Read the model definition and answer for the solid it produces. Units are mm, in the model's axes. A direction names the side the tool comes from. Coordinates: 2 decimals unless noted, no trailing zeros. Write each loop counter-clockwise with the first axis right and the second up, starting at its lowest first coordinate (ties: lowest second). Pieces come first, ordered by that corner, then holes. Notation, with made-up numbers: (67, 28) -> (102, 28) arc R27 ccw to (102, 54) -> close; hole circle Ø3 at (7, 24.25). An arc over 180 degrees is marked (long way). Return JSON: item names as keys, results as strings.
from build123d import *

# Parameters (mm, degrees)
BOSS_EXTRUDE1_DEPTH                     = 55
SHELL1_T                                = -3
CUT_EXTRUDE1_DEPTH                      = 2
BATTERY_CONNECTOR_SKETCH_3_R            = 2.15
CUT_EXTRUDE2_DEPTH                      = 3
BATTERY_CONNECTOR_SKETCH_4_R            = 2.15
CUT_EXTRUDE3_DEPTH                      = 3
BOSS_EXTRUDE6_START                     = 12.75
BOSS_EXTRUDE6_DEPTH                     = 12.75
CONNECTOR_SIDE_MOUNT_SKETCH_R           = 1.55
CONNECTOR_SIDE_MOUNT_SKETCH_R_2         = 1.505
CONNECTOR_MOUNT_PINS_SOCKETS_DEPTH      = 2.4
CONNECTOR_MOUNT_PINS_SOCKETS_SKETCH_3_W = 24.3
CONNECTOR_MOUNT_PINS_SOCKETS_SKETCH_3_H = 1.2
BOSS_EXTRUDE7_DEPTH                     = 0.7
PARTITION_SKETCH_W                      = 3
PARTITION_SKETCH_H                      = 62.75
PARTITION_BOSS_DEPTH                    = 52
SKETCH28_R                              = 3.5
PARTITION_CABLE_PASS_HOLE_DEPTH         = 3
CAVITY2_START                           = 2.577739742
CAVITY2_DEPTH                           = 0.461520646
BOSS_EXTRUDE8_DEPTH                     = 4


# Read off the part's stored shape, not the designer's step: Cavity2
with BuildPart() as part:
    # Sketch2 → Boss-Extrude1 (new body)
    with BuildSketch(Plane(origin=(0, 0, 0), x_dir=(1, 0, 0), z_dir=(0, 1, 0))):
        with BuildLine():
            Line((47.5, -34.375), (-47.5, -34.375))
            ThreePointArc((-47.5, -34.375), (-51.035533906, -32.910533906), (-52.5, -29.375))
            Line((-52.5, -29.375), (-52.5, 29.375))
            ThreePointArc((-52.5, 29.375), (-51.035533906, 32.910533906), (-47.5, 34.375))
            Line((-47.5, 34.375), (47.5, 34.375))
            ThreePointArc((47.5, 34.375), (51.035533906, 32.910533906), (52.5, 29.375))
            Line((52.5, 29.375), (52.5, -29.375))
            ThreePointArc((52.5, -29.375), (51.035533906, -32.910533906), (47.5, -34.375))
        make_face()
    extrude(amount=BOSS_EXTRUDE1_DEPTH)

    # Shell1
    shell1_openings = [part.faces().sort_by_distance(p)[0] for p in [
        (0, 55, 0),
    ]]
    offset(amount=SHELL1_T, openings=shell1_openings, kind=Kind.INTERSECTION)

    # battery_connector_sketch → Cut-Extrude1 (cut)
    with BuildSketch(Plane(origin=(0, 3, 0), x_dir=(1, 0, 0), z_dir=(0, 1, 0))):
        with BuildLine():
            Line((-48.255414742, -4.831437415), (-48.255414742, -29.131437415))
            ThreePointArc((-48.255414742, -29.131437415), (-47.669628305, -30.545650977), (-46.255414742, -31.131437415))
            Line((-46.255414742, -31.131437415), (-40.255414742, -31.131437415))
            ThreePointArc((-40.255414742, -31.131437415), (-38.84120118, -30.545650977), (-38.255414742, -29.131437415))
            Line((-38.255414742, -29.131437415), (-38.255414742, -21.901437415))
            Line((-38.255414742, -21.901437415), (-39.505414742, -20.561437415))
            Line((-39.505414742, -20.561437415), (-39.505414742, -13.401437415))
            Line((-39.505414742, -13.401437415), (-38.255414742, -12.061437415))
            Line((-38.255414742, -12.061437415), (-38.255414742, -4.831437415))
            ThreePointArc((-38.255414742, -4.831437415), (-38.84120118, -3.417223852), (-40.255414742, -2.831437415))
            Line((-40.255414742, -2.831437415), (-46.255414742, -2.831437415))
            ThreePointArc((-46.255414742, -2.831437415), (-47.669628305, -3.417223852), (-48.255414742, -4.831437415))
        make_face()
    extrude(amount=-CUT_EXTRUDE1_DEPTH, mode=Mode.SUBTRACT)

    # battery_connector_sketch<3> → Cut-Extrude2 (cut)
    with BuildSketch(Plane(origin=(0, 3, 0), x_dir=(1, 0, 0), z_dir=(0, 1, 0))):
        with Locations(Location((-43.255414742, -6.881437415, 0), (0, 0, 270))):
            Circle(BATTERY_CONNECTOR_SKETCH_3_R)
    extrude(amount=-CUT_EXTRUDE2_DEPTH, mode=Mode.SUBTRACT)

    # battery_connector_sketch<4> → Cut-Extrude3 (cut)
    with BuildSketch(Plane(origin=(0, 3, 0), x_dir=(1, 0, 0), z_dir=(0, 1, 0))):
        with Locations(Location((-43.255414742, -24.831437415, 0), (0, 0, 270))):
            Circle(BATTERY_CONNECTOR_SKETCH_4_R)
    extrude(amount=-CUT_EXTRUDE3_DEPTH, mode=Mode.SUBTRACT)

    # Sketch25 → Boss-Extrude6 (add)
    with BuildSketch(Plane(origin=(0, 3, 0), x_dir=(1, 0, 0), z_dir=(0, 1, 0)).offset(BOSS_EXTRUDE6_START)):
        with BuildLine():
            Line((-46.255414742, -31.131437415), (-48.456518483, -31.131437415))
            ThreePointArc((-48.456518483, -31.131437415), (-49.21945296, -30.396509431), (-49.5, -29.375))
            Line((-49.5, -29.375), (-49.5, -2.831437415))
            Line((-49.5, -2.831437415), (-46.255414742, -2.831437415))
            ThreePointArc((-46.255414742, -2.831437415), (-47.669628305, -3.417223852), (-48.255414742, -4.831437415))
            Line((-48.255414742, -4.831437415), (-48.255414742, -29.131437415))
            ThreePointArc((-48.255414742, -29.131437415), (-47.669628305, -30.545650977), (-46.255414742, -31.131437415))
        make_face()
    extrude(amount=-BOSS_EXTRUDE6_DEPTH)

    # connector_side_mount_sketch → connector_mount_pins_sockets (cut)
    with BuildSketch(Plane(origin=(-48.255414742, 0, 0), x_dir=(0, 0, -1), z_dir=(1, 0, 0))):
        with Locations((-9.891437415, 11.25)):
            Circle(CONNECTOR_SIDE_MOUNT_SKETCH_R)
        with Locations(Location((-24.071437415, 11.25, 0), (0, 0, 180))):
            Circle(CONNECTOR_SIDE_MOUNT_SKETCH_R_2)
    extrude(amount=-CONNECTOR_MOUNT_PINS_SOCKETS_DEPTH, mode=Mode.SUBTRACT)

    # connector_mount_pins_sockets_sketch<3> → Boss-Extrude7 (add)
    with BuildSketch(Plane(origin=(-48.255414742, 0, 0), x_dir=(0, 0, -1), z_dir=(1, 0, 0))):
        with Locations((-16.981437415, 6.6)):
            Rectangle(CONNECTOR_MOUNT_PINS_SOCKETS_SKETCH_3_W, CONNECTOR_MOUNT_PINS_SOCKETS_SKETCH_3_H)
    extrude(amount=BOSS_EXTRUDE7_DEPTH)

    # partition-sketch → partition-boss (add)
    with BuildSketch(Plane(origin=(0, 3, 0), x_dir=(1, 0, 0), z_dir=(0, 1, 0))):
        with Locations((17.270599113, 0)):
            Rectangle(PARTITION_SKETCH_W, PARTITION_SKETCH_H)
    extrude(amount=PARTITION_BOSS_DEPTH)

    # Sketch28 → partition-cable-pass-hole (cut)
    with BuildSketch(Plane(origin=(18.770599113, 0, 0), x_dir=(0, 0, -1), z_dir=(1, 0, 0))):
        with Locations((26.075, 6.6)):
            Circle(SKETCH28_R)
    extrude(amount=-PARTITION_CABLE_PASS_HOLE_DEPTH, mode=Mode.SUBTRACT)

    # Cavity2 outline → Cavity2 (cut)
    with BuildSketch(Plane(origin=(0, 0, 0), x_dir=(0.9999910167650304, -0.004238677770298889, 0), z_dir=(0.004238677770298889, 0.9999910167650305, 0)).offset(CAVITY2_START)):
        Polygon((0.430972634, 22.782282347), (9.255972634, 22.782282347), (9.255972634, 29.062282347), (-9.594027366, 29.062282347), (-9.594027366, 22.782282347), (-0.769027366, 22.782282347), (-2.890347709, 20.660962004), (-0.769027366, 18.53964166), (-9.594027366, 18.53964166), (-9.594027366, 12.25964166), (9.255972634, 12.25964166), (9.255972634, 18.53964166), (0.430972634, 18.53964166), (2.552292978, 20.660962004), align=None)
        Polygon((-0.169027366, 18.53964166), (-2.290347709, 20.660962004), (-0.169027366, 22.782282347), (1.952292978, 20.660962004), align=None, mode=Mode.SUBTRACT)
    extrude(amount=CAVITY2_DEPTH, mode=Mode.SUBTRACT)

    # Sketch32 → Boss-Extrude8 (add)
    with BuildSketch(Plane(origin=(0, 3, 0), x_dir=(1, 0, 0), z_dir=(0, 1, 0))):
        Polygon((-0.144808067, 22.60955262), (1.795970783, 20.66877377), (-0.144808067, 18.727994921), (-2.085586916, 20.66877377), align=None)
    extrude(amount=BOSS_EXTRUDE8_DEPTH)


solid = part.part
1. For a pull along Y with two mould halves and no side action, classify faces 1 (the face through (17.29, 5.26, -29.31)), 2 (the face through (34, 3, 0)), 3 (the face through (51.074, 27.115, 32.871)) as +Y half, -Y half, draft (parallel to the pull), parting line (faces both ways), or undercut.
Taken from the geometry:
{"face 1": "undercut", "face 2": "+Y half", "face 3": "draft"}
2. The part is cut by section B-B (x = -26). Determine the outline of the cut face in (y, z) (3 decimals), then the cut area to 3 significant figures.
Taken from the geometry:
{"outline": "(0, -34.375) -> (55, -34.375) -> (55, -31.375) -> (3, -31.375) -> (3, 31.375) -> (55, 31.375) -> (55, 34.375) -> (0, 34.375) -> close", "area": "518 mm2"}
3. The part is cut by section C-C (z = -27). Determine the outline of the cut face in (x, y), then the cut area to 3 significant figures.
Taken from the geometry:
{"outline": "(-52.5, 0) -> (52.5, 0) -> (52.5, 55) -> (49.5, 55) -> (49.5, 3) -> (18.77, 3) -> (18.77, 3.22) -> (15.77, 3.22) -> (15.77, 3) -> (9.27, 3) -> (9.27, 2.54) -> (-9.58, 2.62) -> (-9.58, 3) -> (-49.5, 3) -> (-49.5, 55) -> (-52.5, 55) -> close; (15.77, 9.98) -> (18.77, 9.98) -> (18.77, 55) -> (15.77, 55) -> close", "area": "755 mm2"}
4. The part is cut by section D-D (z = -6.5). Determine the outline of the cut face in (x, y), then the cut area to 3 significant figures.
Taken from the geometry:
{"outline": "(-52.5, 0) -> (52.5, 0) -> (52.5, 55) -> (49.5, 55) -> (49.5, 3) -> (18.77, 3) -> (18.77, 55) -> (15.77, 55) -> (15.77, 3) -> (-49.5, 3) -> (-49.5, 55) -> (-52.5, 55) -> close", "area": "783 mm2"}
5. The part is cut by section A-A (y = 11.25). Count the separate pieces of the cut face and the enclosed holes in it, then the cut area to 3 significant figures.
Taken from the geometry:
{"separate pieces": "1", "enclosed holes": "2", "area": "1,200 mm2"}
6. Flat-ended cylindrical pins translate along their axes: pin 1 Ø4 at (x, z) = (29.5, -8) entering from +Y; pin 2 Ø4.5 at (x, z) = (0, -21.5) entering from +Y. Find the tip coordinate at first contact, or state that the pin passes through.
Taken from the geometry:
{"pin 1": "stops at y = 3", "pin 2": "stops at y = 7"}
7. Consider L1, parallel to X at y = 44, z = -6.5; L2, parallel to Z at x = -28, y = 11 (3 decimals); L3, parallel to Z at x = -48, y = 11. Determine where each line is inside the solid, lowest interval first.
Taken from the geometry:
{"L1": "x = -52.5 to -49.5, 15.77 to 18.77, 49.5 to 52.5", "L2": "z = -34.375 to -31.375, 31.375 to 34.375", "L3": "z = -34.35 to -31.31, 2.83 to 3.85, 30.11 to 31.13, 31.31 to 34.35"}
8. A tool of negligible diameter and unlimited length cuts with its end or side. For faces 4 (the face through (-1, 27, -34.375)), 5 (the face through (-49.439, 10.233, 22.962)), 6 (the face through (15.771, 29, 0)), from which of +Z, -Z, +X, -X, +Y, -Y can it reach the whole face along a straight path? Write none if from no direction.
Taken from the geometry:
{"face 4": "-Z, +X, -X, +Y, -Y", "face 5": "none", "face 6": "+Y"}
